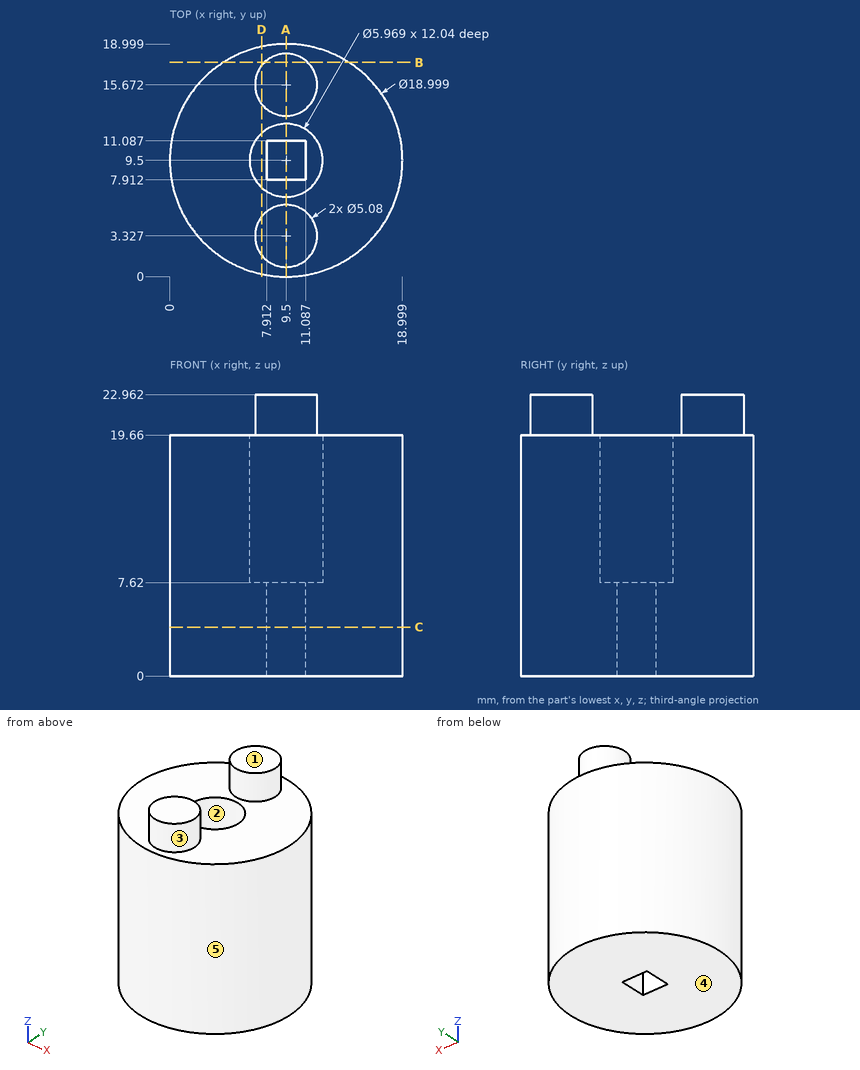
Could you check a few things on this drawing? It's one solid part, dimensions in mm from its lowest x, y, z. A direction names the side the tool comes from. Round coordinates to 2 decimals unless told otherwise and drop trailing zeros. Loops run counter-clockwise (first coordinate to the right, second up) from the corner with the lowest first, then second, coordinate; pieces in that order, holes last. Notation, with made-up numbers: (81, 32.5) -> (130, 32.5) arc R20 ccw to (130, 59.5) -> close; hole circle Ø1 at (58, -25). An arc over 180 degrees is marked (long way). One line per item, written item: value. Start each with the question number.
1. If we section it at B-B, the plane y = 17.5: Write out the boundary of the cut face in (x, z).
2. For pin 1 (4 mm diameter, centred on x = 3.5, y = 8.5, fed in from +Z); pin 2 (2 mm diameter, centred on x = 6.5, z = 12, fed in from -Y); pin 3 (8 mm diameter, centred on y = 10.5, z = 19, fed in from -X); pin 4 (1 mm diameter, centred on y = 17, z = 14, fed in from -X), each with a flat end and sliding along its axis, tell me the tip position at first contact or that it passes through.
3. If we mould it in two halves opening along Y, with no side actions, what happens to the marked faces 3, 4 and 5? For each: pulls with the +Y half, pulls with the -Y half, needs draft (parallel to the pull), parting line crosses it, or undercut.
4. For the marked faces 1 and 2, which set-ups out of +Z, -Z, +X, -X, +Y, -Y let a thin tool reach every point of the face, with its end or its side?
5. If we section it at A-A, the plane x = 9.5: Write out the boundary of the cut face in (y, z) (1 decimal), then the cut area to 3 significant figures.
6. If we section it at D-D, the plane x = 7.5: Write out the boundary of the cut face in (y, z) (1 decimal).
7. If I drill on probe 1 along X at (y, z) = (11, 5.5); probe 2 along Z at (x, y) = (13, 16.75); probe 3 along X at (y, z) = (8, 7.75), over which ranges is the centre line in solid material (lowest first)?
8. If we section it at C-C, the plane z = 4: Write out the boundary of the cut face in (x, y).
Calculated:
1. outline: (4.38, 0) -> (14.62, 0) -> (14.62, 19.66) -> (11.26, 19.66) -> (11.26, 22.96) -> (7.74, 22.96) -> (7.74, 19.66) -> (4.38, 19.66) -> close
2. pin 1: stops at z = 19.66
2. pin 2: stops at y = 0.21
2. pin 3: stops at x = 0
2. pin 4: stops at x = 3.08
3. face 3: undercut
3. face 4: needs draft
3. face 5: parting line crosses it
4. face 1: +Z, +X, -X, +Y, -Y
4. face 2: +Z
5. outline: (0, 0) -> (7.9, 0) -> (7.9, 7.6) -> (6.5, 7.6) -> (6.5, 19.7) -> (5.9, 19.7) -> (5.9, 23) -> (0.8, 23) -> (0.8, 19.7) -> (0, 19.7) -> close; (11.1, 0) -> (19, 0) -> (19, 19.7) -> (18.2, 19.7) -> (18.2, 23) -> (13.1, 23) -> (13.1, 19.7) -> (12.5, 19.7) -> (12.5, 7.6) -> (11.1, 7.6) -> close
5. area: 311 mm²
6. outline: (0.2, 0) -> (18.8, 0) -> (18.8, 19.7) -> (17.2, 19.7) -> (17.2, 23) -> (14.1, 23) -> (14.1, 19.7) -> (11.7, 19.7) -> (11.7, 7.6) -> (7.3, 7.6) -> (7.3, 19.7) -> (4.9, 19.7) -> (4.9, 23) -> (1.8, 23) -> (1.8, 19.7) -> (0.2, 19.7) -> close
7. probe 1: x = 0.12 to 7.91, 11.09 to 18.88
7. probe 2: z = 0 to 19.66
7. probe 3: x = 0.12 to 6.92, 12.08 to 18.88
8. outline: circle Ø19 at (9.5, 9.5); hole (7.91, 7.91) -> (11.09, 7.91) -> (11.09, 11.09) -> (7.91, 11.09) -> close
